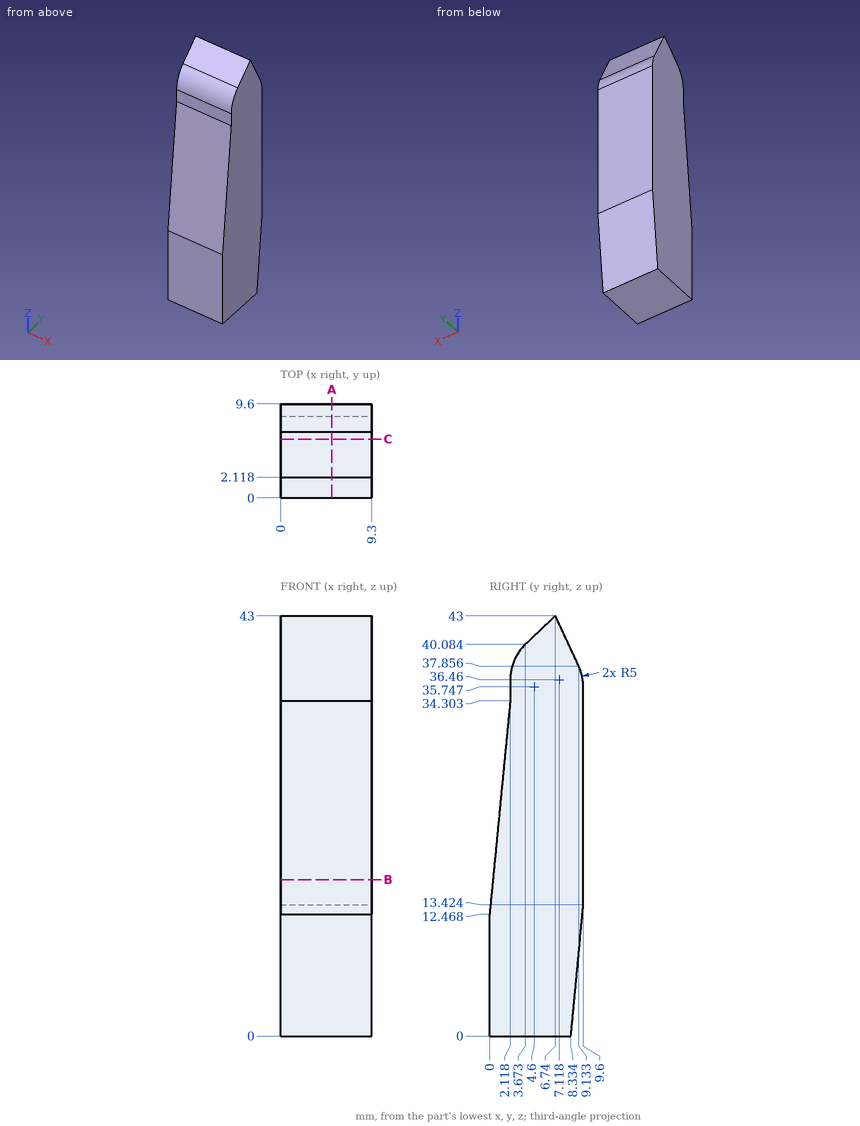
Input: dimensioned drawing with shaded views. Units: mm. Origin: part minimum x, y, z. Coordinates: 2 decimals unless noted, no trailing zeros. Write each loop counter-clockwise with the first axis right and the second up, starting at its lowest first coordinate (ties: lowest second). Pieces come first, ordered by that corner, then holes. Notation, with made-up numbers: M 87,74 L 123,74 A17 cw 123,79 Z; hole C 33.25,-23.5 d8. An arc over 180 degrees is marked long. Answer as CSV lines item,"result". Start each with the question number.
Q1. Cut plane A-A on x = 5.25. Return the cut outline in (y, z) (1 decimal), then the cut area to 3 significant figures.
Q2. Cut plane B-B on z = 16. Return the cut outline in (x, y), then the cut area to 3 significant figures.
Q3. Cut plane C-C on y = 6. Return the cut outline in (x, z), then the cut area to 3 significant figures.
Q4. Pin query (flat end, axial travel): P1, Ø2, axis at x = 2, z = 20, coming from the -Y side; P2, Ø3, axis at x = 4, z = 11, coming from the +Y side; P3, Ø2.5, axis at x = 6.5, z = 35, coming from the -Y side. Return the tip coordinate at first contact, or that it passes through.
Q5. Line query: line 1 (Z direction, x = 8, y = 7.75) (1 decimal); line 2 (Z direction, x = 7, y = 6) (1 decimal); line 3 (Y direction, x = 2.75, z = 25) (1 decimal). Output: solid intervals per line, ascending. Write a range as from..to.
Findings below:
1,outline,"M 0,0 L 8.3,0 L 9.6,13.4 L 9.6,35.7 A5 ccw 9.1,37.9 L 6.7,43 L 3.7,40.1 A5 ccw 2.1,36.5 L 2.1,34.3 L 0,12.5 Z"
1,area,"343 mm2"
2,outline,"M 0,0.34 L 9.3,0.34 L 9.3,9.6 L 0,9.6 Z"
2,area,"86.1 mm2"
3,outline,"M 0,0 L 9.3,0 L 9.3,42.3 L 0,42.3 Z"
3,area,"393 mm2"
4,P1,"stops at y = 0.63"
4,P2,"stops at y = 9.51"
4,P3,"stops at y = 2.06"
5,line 1,"z = 0..40.8"
5,line 2,"z = 0..42.3"
5,line 3,"y = 1.2..9.6"
